```python
from build123d import *

# Parameters (mm, degrees)
SKETCH1_W           = 80
SKETCH1_H           = 110
BOSS_EXTRUDE1_DEPTH = 3
D_GAGEMENT_M41_D    = 4.5


with BuildPart() as part:
    # Sketch1 → Boss-Extrude1 (new body)
    with BuildSketch(Plane.XY):
        Rectangle(SKETCH1_W, SKETCH1_H)
    extrude(amount=BOSS_EXTRUDE1_DEPTH)

    # Dégagement M41 (through all)
    with Locations(Plane.XY.offset(3)):
        with Locations((27.50000229, 47.500001598), (27.50000229, 8.500001598), (-27.49999771, 8.500001598), (-27.49999771, 47.500001598)):
            Hole(D_GAGEMENT_M41_D / 2)


solid = part.part
```
The listing builds one solid part. Answer for the finished solid, in the listing's coordinates (mm). Round coordinates to 2 decimals unless told otherwise and drop trailing zeros. Write each loop counter-clockwise with the first axis right and the second up, starting at its lowest first coordinate (ties: lowest second). Pieces come first, ordered by that corner, then holes. Notation, with made-up numbers: (-33.75, 49.5) -> (-14.75, 49.5) arc R3 cw to (-14.75, 54.5) -> close; hole circle Ø2 at (-21, 15.25). An arc over 180 degrees is marked (long way). Write item = value, one per line.
1) Section A-A on x = 28 is taken. Write down the section's boundary in (y, z).
Check values:
outline = (-55, 0) -> (6.31, 0) -> (6.31, 3) -> (-55, 3) -> close; (10.69, 0) -> (45.31, 0) -> (45.31, 3) -> (10.69, 3) -> close; (49.69, 0) -> (55, 0) -> (55, 3) -> (49.69, 3) -> close
2) Straight lines are drawn through the part: line 1 along Y through (x, z) = (-27.5, 1.7); line 2 along X through (y, z) = (47, 2.4); line 3 along Y through (x, z) = (26, 1.35). For each, find the intervals that lie inside material, in ascending order. Write a range as [from, to].
Check values:
line_1 = [-55, 6.25], [10.75, 45.25], [49.75, 55]
line_2 = [-40, -29.69], [-25.31, 25.31], [29.69, 40]
line_3 = [-55, 6.82], [10.18, 45.82], [49.18, 55]
3) Given pin 1 (6 mm diameter, centred on x = -28, y = 10, fed in from -Z), flat-ended and moving along its own axis, determine where the tip first touches the part or whether it passes through.
Check values:
pin_1 = 0
4) For a pull along Y with two mould halves and no side action, classify faces 1 (the flat face through (-1, 1, 3)), 2 (the cylindrical face through (26.29, 49.397, 1.479)), 3 (the flat face through (-1, 55, 1)) as released by +Y, released by -Y, zero draft, split by the parting line, or undercut.
Check values:
face_1 = zero draft
face_2 = undercut
face_3 = released by +Y
